Verification items for the finished model (mm, model axes). A direction names the side the tool comes from. Give positions to 0.01 mm unless a question says otherwise; leave off trailing zeros. Order: outer loops, then holes, each group sorted by start corner. A loop starts at its lowest first (then second) coordinate and runs counter-clockwise, first axis right, second up. Notation, with made-up numbers: (-6, 57) - (14, 57) arc R26 ccw to (14, 79) - close; hole circle Ø10 at (50.25, -36). An arc over 180 degrees is marked (long way). Answer as a JSON object with one key per item and string values. Group by question number.
(1) Depth check by flat-ended pin: pin 1 Ø6 at (y, z) = (-12, -8.5) entering from +X; pin 2 Ø1.8 at (x, y) = (15, -9) entering from -Z; pin 3 Ø14.5 at (x, y) = (0, 0) entering from +Z. Enter the tip coordinate at first touch or a pass-through.
(2) Section check B-B (x = 0). Record the boundary of the cut face in (y, z) (1 decimal), then the cut area to 3 significant figures.
(3) Section check D-D (y = -12.5). Record the boundary of the cut face in (x, z), then the cut area to 3 significant figures.
(4) Access from +Z, -Z, +X, -X, +Y, -Y to the whole of each face (thin tool, end or side, straight path). Record for faces 1 (the face through (-15, -9, -8)), 2 (the face through (3.441, -15.497, -6.084)), 3 (the face through (2.5, 18, -4)).
(5) Section check A-A (y = 0). Record the boundary of the cut face in (x, z) (1 decimal), then the cut area to 3 significant figures.
(6) Thickness scan on line 1 (X direction, y = 0, z = -12.25); line 2 (X direction, y = 0, z = -3.3) (3 decimals). Record the ranges inside material, lowest first.
(7) Section check C-C (z = -5.5). Record the boundary of the cut face in (x, y) (3 decimals), then the cut area to 3 significant figures.
(8) Mould release check, pull along X, two halves, no side actions. Record for faces 4 (the face through (14.034, -10.99, -3.944)), 5 (the face through (-17.023, -9.869, -3.944)), 6 (the face through (0, -3, -17)): +X half, -X half, draft (parallel to the pull), parting line (faces both ways), or undercut.
```python
from build123d import *

# Parameters (mm, degrees)
F3_D           = 5
F3_CBORE_D     = 16
F3_CBORE_DEPTH = 6
F4_W           = 5
F4_H           = 4
F5_DEPTH       = 8
F6_COUNT       = 3


with BuildPart() as f1:
    # F0 (on Front) → F1 (revolve)
    with BuildSketch(Plane.XZ):
        Polygon((0, -17), (0, 0), (-15.875, 0), (-15.875, -12), (-14.2875, -12), (-14.2875, -17), align=None)
    revolve(axis=Axis((0, 0, -23.116006), (0, 0, -1)))

    # F3 (through all)
    with Locations(Plane.XY):
        with Locations((0, 0)):
            CounterBoreHole(F3_D / 2, F3_CBORE_D / 2, F3_CBORE_DEPTH)

    # F4 (on face) → F5 (join)
    with BuildSketch(Plane.XY):
        with Locations((0, 17.676914)):
            Rectangle(F4_W, F4_H)
    extrude(amount=-F5_DEPTH)

    # F6: F1 ×3 about axis
    f6_axis = Axis((0, 0, -12), (0, 0, -1))


with BuildPart() as f1_1:
    add(f1.part)
    for i in range(1, F6_COUNT):
        add(f1.part.rotate(f6_axis, i * 360 / F6_COUNT))


solid = f1_1.part
```
Solutions:
{
 "1": {"pin 1": "stops at x = 17.5", "pin 2": "stops at z = -8", "pin 3": "stops at z = -6"},
 "2": {"outline": "(-15.9, -12) - (-14.3, -12) - (-14.3, -17) - (-2.5, -17) - (-2.5, -6) - (-8, -6) - (-8, 0) - (-15.9, 0) - close; (2.5, -17) - (14.3, -17) - (14.3, -12) - (15.9, -12) - (15.9, -8) - (19.7, -8) - (19.7, 0) - (8, 0) - (8, -6) - (2.5, -6) - close", "area": "403 mm2"},
 "3": {"outline": "(-9.79, -12) - (-6.92, -12) - (-6.92, -17) - (6.92, -17) - (6.92, -12) - (9.79, -12) - (9.79, 0) - (-9.79, 0) - close", "area": "304 mm2"},
 "4": {"face 1": "-Z, -X, -Y", "face 2": "-Z", "face 3": "+Z, -Z, +X, +Y"},
 "5": {"outline": "(-15.9, -12) - (-14.3, -12) - (-14.3, -17) - (-2.5, -17) - (-2.5, -6) - (-8, -6) - (-8, 0) - (-15.9, 0) - close; (2.5, -17) - (14.3, -17) - (14.3, -12) - (15.9, -12) - (15.9, 0) - (8, 0) - (8, -6) - (2.5, -6) - close", "area": "373 mm2"},
 "6": {"line 1": "x = -14.29 to -2.5, 2.5 to 14.29", "line 2": "x = -15.875 to -8, 8 to 15.875"},
 "7": {"outline": "(-18.291, -7.673) - (-15.791, -12.004) - (-12.327, -10.004) arc R15.875 ccw to (12.327, -10.004) - (15.791, -12.004) - (18.291, -7.673) - (14.827, -5.673) arc R15.875 ccw to (2.5, 15.677) - (2.5, 19.677) - (-2.5, 19.677) - (-2.5, 15.677) arc R15.875 ccw to (-14.827, -5.673) - close; hole circle Ø16 at (0, 0)", "area": "649 mm2"},
 "8": {"face 4": "undercut", "face 5": "-X half", "face 6": "draft"}
}
